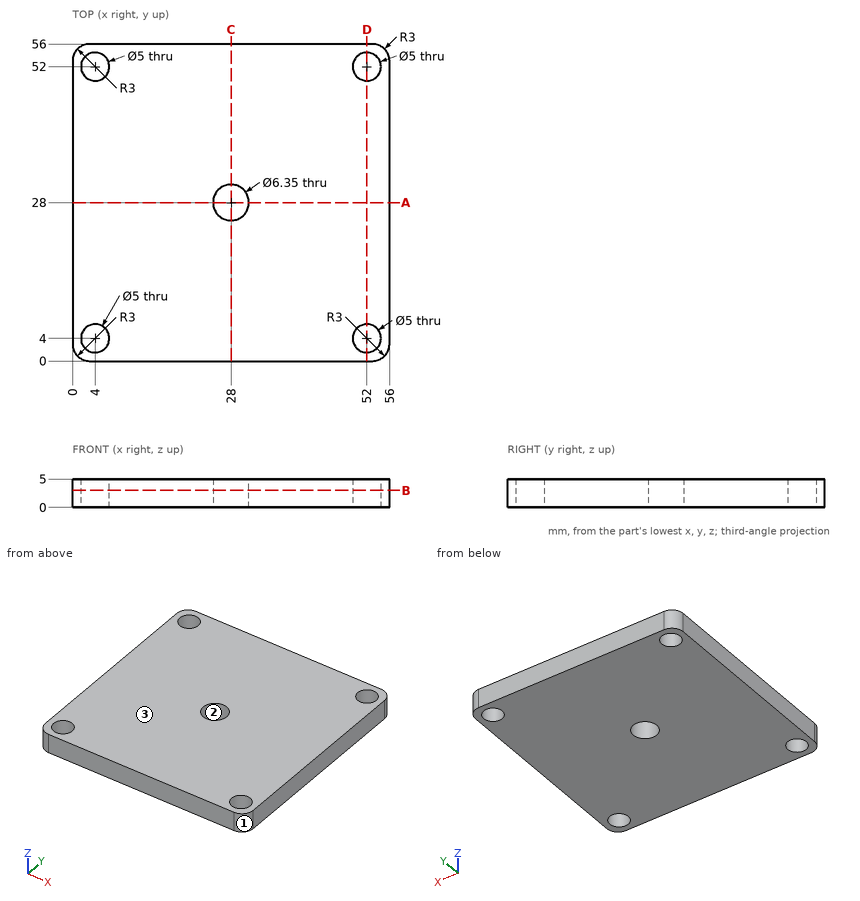
The figure shows three views and two pictorial views of one solid part (mm, origin at its lowest corner). Answer the questions. Give positions to 0.01 mm unless a question says otherwise; leave off trailing zeros. Write each loop counter-clockwise with the first axis right and the second up, starting at its lowest first coordinate (ties: lowest second). Pieces come first, ordered by that corner, then holes. Notation, with made-up numbers: (-25.5, 2.5) - (-7.5, 2.5) arc R25 cw to (-7.5, 30.5) - close; hole circle Ø8 at (72.5, 5). An arc over 180 degrees is marked (long way). Return JSON: item names as keys, results as strings.
Q1. For a pull along X with two mould halves and no side action, classify the marked faces 1, 2 and 3 as released by +X, released by -X, zero draft, split by the parting line, or undercut.
Reply:
{"face 1": "released by +X", "face 2": "undercut", "face 3": "zero draft"}
Q2. A cutting plane is placed at A-A, the plane y = 28. Determine the outline of the cut face in (x, z) (3 decimals), and give its area (3 significant figures).
Reply:
{"outline": "(0, 0) - (24.825, 0) - (24.825, 5) - (0, 5) - close; (31.175, 0) - (56, 0) - (56, 5) - (31.175, 5) - close", "area": "248 mm²"}
Q3. Consider line 1 along Y through (x, z) = (52, 2.55); line 2 along X through (y, z) = (3, 1.3). Determine where each line is inside the solid, lowest interval first. Write a range as [from, to].
Reply:
{"line 1": "[0, 1.5], [6.5, 49.5], [54.5, 56]", "line 2": "[0, 1.71], [6.29, 49.71], [54.29, 56]"}
Q4. A cutting plane is placed at D-D, the plane x = 52. Determine the outline of the cut face in (y, z), and give its area (3 significant figures).
Reply:
{"outline": "(0, 0) - (1.5, 0) - (1.5, 5) - (0, 5) - close; (6.5, 0) - (49.5, 0) - (49.5, 5) - (6.5, 5) - close; (54.5, 0) - (56, 0) - (56, 5) - (54.5, 5) - close", "area": "230 mm²"}
Q5. A cutting plane is placed at B-B, the plane z = 3. Determine the outline of the cut face in (x, y) (3 decimals), and give its area (3 significant figures).
Reply:
{"outline": "(0, 3) arc R3 ccw to (3, 0) - (53, 0) arc R3 ccw to (56, 3) - (56, 53) arc R3 ccw to (53, 56) - (3, 56) arc R3 ccw to (0, 53) - close; hole circle Ø5 at (4, 4); hole circle Ø5 at (4, 52); hole circle Ø6.35 at (28, 28); hole circle Ø5 at (52, 4); hole circle Ø5 at (52, 52)", "area": "3,020 mm²"}
